```python
from build123d import *

# Parameters (mm, degrees)
SKETCH1_W           = 101.6
SKETCH1_H           = 101.6
SKETCH1_R           = 3.856433765
SKETCH1_R_2         = 6.35
BOSS_EXTRUDE1_DEPTH = 3
SKETCH1_4_R         = 6.35
BOSS_EXTRUDE2_DEPTH = 203.2


with BuildPart() as part:
    # Sketch1 → Boss-Extrude1 (new body)
    # profile 1 of 2: a face of its own
    with BuildSketch(Plane.XY):
        Rectangle(SKETCH1_W, SKETCH1_H)
        with Locations((38.1, 38.1)):
            Circle(SKETCH1_R, mode=Mode.SUBTRACT)
        with Locations((-38.1, 38.1)):
            Circle(SKETCH1_R, mode=Mode.SUBTRACT)
        Circle(SKETCH1_R_2, mode=Mode.SUBTRACT)
        with Locations((38.1, -38.1)):
            Circle(SKETCH1_R, mode=Mode.SUBTRACT)
        with Locations((-38.1, -38.1)):
            Circle(SKETCH1_R, mode=Mode.SUBTRACT)
    # profile 2 of 2: a face of its own
    with BuildSketch(Plane.XY):
        Circle(SKETCH1_R_2)
    extrude(amount=BOSS_EXTRUDE1_DEPTH)

    # Sketch1_4 → Boss-Extrude2 (add)
    with BuildSketch(Plane.XY):
        Circle(SKETCH1_4_R)
    extrude(amount=-BOSS_EXTRUDE2_DEPTH)


solid = part.part
```
Can you work these out from the model? Positions are in its coordinate system, mm. Round coordinates to 2 decimals unless told otherwise and drop trailing zeros. Loops run counter-clockwise (first coordinate to the right, second up) from the corner with the lowest first, then second, coordinate; pieces in that order, holes last. Notation, with made-up numbers: M 58,78.5 L 63,78.5 A19 cw 63,102.5 Z; hole C -25.5,15 d6. An arc over 180 degrees is marked long. Answer in a Markdown table with one row per item.
1. If we section it at C-C, the plane x = 0: Please give me the cut outline in (y, z).
Established:
| item | result |
|---|---|
| outline | M -50.8,0 L -6.35,0 L -6.35,-203.2 L 6.35,-203.2 L 6.35,0 L 50.8,0 L 50.8,3 L -50.8,3 Z |
2. I'm going to push flat-ended pins straight in: pin 1 Ø1.5 at (x, z) = (-6, -125) entering from +Y; pin 2 Ø9 at (x, y) = (-38.1, 38.1) entering from -Z. Where does each tip first touch, or does it pass through?
Established:
| item | result |
|---|---|
| pin 1 | y = 3.57 |
| pin 2 | z = 0 |
3. If we section it at D-D, the plane y = -15: Please give me the cut outline in (x, z), plus the area to 3 significant figures.
Established:
| item | result |
|---|---|
| outline | M -50.8,0 L 50.8,0 L 50.8,3 L -50.8,3 Z |
| area | 305 mm² |
4. Please list where these lines run through material, in increasing order: line 1 (Y direction, x = -38, z = 1); line 2 (Z direction, x = -45.5, y = 14); line 3 (Y direction, x = -2, z = -85). Write a range as from..to.
Established:
| item | result |
|---|---|
| line 1 | -50.8..-41.96, -34.24..34.24, 41.96..50.8 |
| line 2 | 0..3 |
| line 3 | -6.03..6.03 |
5. If we section it at A-A, the plane y = -38.1: Please give me the cut outline in (x, z), plus the area to 3 significant figures.
Established:
| item | result |
|---|---|
| outline | M -50.8,0 L -41.96,0 L -41.96,3 L -50.8,3 Z; M -34.24,0 L 34.24,0 L 34.24,3 L -34.24,3 Z; M 41.96,0 L 50.8,0 L 50.8,3 L 41.96,3 Z |
| area | 259 mm² |
6. Thinking about a two-plate mould opening in Y: for faces 1 (the face through (-1.38, -6.2, -100.18)), 2 (the face through (-34.54, 36.62, 1.48)), 3 (the face through (-1, 1, 3)), which applies, pulls with the +Y half, pulls with the -Y half, needs draft (parallel to the pull), parting line crosses it, or undercut?
Established:
| item | result |
|---|---|
| face 1 | parting line crosses it |
| face 2 | undercut |
| face 3 | needs draft |
